```python
from build123d import *

# Parameters (mm, degrees)
F1_DEPTH      = 44.45
F2_W          = 73.025
F2_H          = 65.0875
F3_DEPTH      = 28.576
F3_DEPTH_BACK = 28.576
F4_R          = 9.92251
F5_DEPTH      = 88.901
F7_DEPTH      = 7.9375
F8_R          = 10.3251
F9_DEPTH      = 7.9385
F10_R         = 6.35
F11_R         = 12.7


with BuildPart() as f1:
    # F0 (on Front) → F1 (new body, symmetric)
    with BuildSketch(Plane.XZ):
        with BuildLine():
            Line((-28.575, 44.45), (-28.575, 0))
            Line((-28.575, 0), (28.575, 0))
            Line((28.575, 0), (28.575, 44.45))
            ThreePointArc((28.575, 44.45), (0, 73.025), (-28.575, 44.45))
        make_face()
    extrude(amount=F1_DEPTH, both=True)

    # F2 (on Right) → F3 (cut, two sides)
    with BuildSketch(Plane.YZ) as f3_sk:
        with Locations((0, 40.48125)):
            Rectangle(F2_W, F2_H)
    extrude(amount=-F3_DEPTH, mode=Mode.SUBTRACT)
    extrude(f3_sk.sketch, amount=F3_DEPTH_BACK, mode=Mode.SUBTRACT)

    # F4 (on face) → F5 (cut, through all)
    with BuildSketch(Plane.XZ.offset(44.45)):
        with Locations((0, 44.45)):
            Circle(F4_R)
    extrude(amount=-F5_DEPTH, mode=Mode.SUBTRACT)

    # F6 (on Top) → F7 (join)
    with BuildSketch(Plane.XY):
        with BuildLine():
            Line((80.01, 22.225), (28.575, 22.225))
            Line((28.575, 22.225), (28.575, -22.225))
            Line((28.575, -22.225), (80.01, -22.225))
            ThreePointArc((80.01, -22.225), (102.235, 0), (80.01, 22.225))
        make_face()
    extrude(amount=F7_DEPTH)

    # F8 (on face) → F9 (cut, through all)
    with BuildSketch(Plane.XY.offset(7.9375)):
        with Locations((41.91, 0)):
            Circle(F8_R)
        with Locations((80.01, 0)):
            Circle(F8_R)
    extrude(amount=-F9_DEPTH, mode=Mode.SUBTRACT)

    # F10
    f10_edges = [f1.edges().sort_by_distance(p)[0] for p in [
        (28.575, -22.225, 3.96875),
        (28.575, 22.225, 3.96875),
    ]]
    fillet(f10_edges, radius=F10_R)

    # F11
    f11_edges = [f1.edges().sort_by_distance(p)[0] for p in [
        (0, -36.5125, 7.9375),
        (0, 36.5125, 7.9375),
        (0, -44.45, 0),
        (0, 44.45, 0),
    ]]
    fillet(f11_edges, radius=F11_R)


solid = f1.part
```
The listing builds one solid part. Answer for the finished solid, in the listing's coordinates (mm). A direction names the side the tool comes from. Give positions to 0.01 mm unless a question says otherwise; leave off trailing zeros. Order: outer loops, then holes, each group sorted by start corner. A loop starts at its lowest first (then second) coordinate and runs counter-clockwise, first axis right, second up. Notation, with made-up numbers: (-0.75, -1.75) -> (12.25, -1.75) arc R13 ccw to (12.25, 13.25) -> close; hole circle Ø5 at (-38.75, 4.5). An arc over 180 degrees is marked (long way). One line per item, written item: value.
1) Determine the mould class of faces 6 (the flat face through (28.575, -38, 22)), 7 (the cylindrical face through (1.49, -32.693, 11.559)), 8 (the cylindrical face through (-2.151, -40.537, 34.763)) for opening direction X: pulls with the +X half, pulls with the -X half, needs draft (parallel to the pull), parting line crosses it, or undercut.
Reported:
face 6: pulls with the +X half
face 7: needs draft
face 8: undercut
2) Find section A-A, the plane x = 41.91. Determine the outline of the cut face in (y, z) (1 decimal).
Reported:
outline: (-22.2, 0) -> (-10.3, 0) -> (-10.3, 7.9) -> (-22.2, 7.9) -> close; (10.3, 0) -> (22.2, 0) -> (22.2, 7.9) -> (10.3, 7.9) -> close
3) Find section B-B, the plane z = 40. Count the separate pieces of the cut face and the enclosed holes in it, plus the area to 3 significant figures.
Reported:
separate pieces: 4
enclosed holes: 0
area: 626 mm^2
4) A tool of negligible diameter and unlimited length cuts with its end or side. For faces 1 (the flat face through (57, -22.225, 4)), 2 (the flat face through (21, 0, 0)), 3 (the cylindrical face through (1.49, 32.693, 11.559)), 4 (the cylindrical face through (0.63, 40.43, 73.02)), 5 (the flat face through (28.575, 38, 17)), from which of +Z, -Z, +X, -X, +Y, -Y can it reach the whole face along a straight path? Write none if from no direction.
Reported:
face 1: +Z, -Z, +X, -Y
face 2: -Z, +X, -X, +Y, -Y
face 3: +Z, +X, -X
face 4: +Z, +Y, -Y
face 5: +Z, -Z, +X, +Y
5) Find section D-D, the plane x = 82. Determine the outline of the cut face in (y, z), plus the area to 3 significant figures.
Reported:
outline: (-22.14, 0) -> (-10.13, 0) -> (-10.13, 7.94) -> (-22.14, 7.94) -> close; (10.13, 0) -> (22.14, 0) -> (22.14, 7.94) -> (10.13, 7.94) -> close
area: 191 mm^2
6) Flat-ended cylindrical pins translate along their axes: P1, Ø14.5, axis at x = 11, y = -6.5, coming from the +Z side; P2, Ø2.5, axis at x = 68.5, z = 4, coming from the +Y side (3 decimals); P3, Ø6, axis at x = -3.5, y = -27.5, coming from the +Z side. Find the tip coordinate at first contact, or state that the pin passes through.
Reported:
P1: stops at z = 7.94
P2: stops at y = 22.225
P3: stops at z = 9.84
7) Find the intervals of material crossed by line 1 (X direction, y = 39, z = 44) (3 decimals); line 2 (Y direction, x = 10, z = 23.5); line 3 (Y direction, x = 80.01, z = 6) (3 decimals), in increasing order.
Reported:
line 1: x = -28.575 to -9.912, 9.912 to 28.575
line 2: y = -44.45 to -36.51, 36.51 to 44.45
line 3: y = -22.225 to -10.325, 10.325 to 22.225
